from build123d import *

# Parameters (mm, degrees)
F0_R      = 3.25
F1_DEPTH  = 2.5
F2_R      = 1.5
F3_DEPTH  = 2.5
F4_R      = 7
F4_R_2    = 1.5
F5_DEPTH  = 3
F6_R      = 1.5
F7_DEPTH  = 3
F8_W      = 2
F8_H      = 2
F9_DEPTH  = 2
F11_DEPTH = 1


with BuildPart() as f1:
    # F0 (on Top) → F1 (new body)
    with BuildSketch(Plane.XY):
        with Locations((-13.149204, -17.084545)):
            Circle(F0_R)
    extrude(amount=F1_DEPTH)

    # F2 (on face) → F3 (join)
    with BuildSketch(Plane.XY.offset(2.5)):
        with Locations((-13.149204, -17.084545)):
            Circle(F2_R)
    extrude(amount=F3_DEPTH)

    # F4 (on face) → F5 (join)
    with BuildSketch(Plane.XY.offset(5)):
        with Locations((-13.149204, -17.084545)):
            Circle(F4_R)
        with Locations((-13.149204, -17.084545)):
            Circle(F4_R_2, mode=Mode.SUBTRACT)
    extrude(amount=F5_DEPTH)

    # F6 (on face) → F7 (join)
    with BuildSketch(Plane.XY.offset(5)):
        with Locations((-13.149204, -17.084545)):
            Circle(F6_R)
    extrude(amount=F7_DEPTH)

    # F8 (on face) → F9 (join)
    with BuildSketch(Plane.XY.offset(8)):
        with Locations((-16.149204, -14.084545)):
            Rectangle(F8_W, F8_H)
        with Locations((-10.149204, -14.084545)):
            Rectangle(F8_W, F8_H)
        with Locations((-10.149204, -20.084545)):
            Rectangle(F8_W, F8_H)
        with Locations((-16.149204, -20.084545)):
            Rectangle(F8_W, F8_H)
    extrude(amount=F9_DEPTH)

    # F10 (on face) → F11 (join)
    with BuildSketch(Plane.XY.offset(10)):
        Polygon((-9.149204, -13.084545), (-15.149204, -13.084545), (-15.149204, -15.084545), (-17.149204, -15.084545), (-17.149204, -21.084545), (-9.149204, -21.084545), align=None)
    extrude(amount=-F11_DEPTH)


solid = f1.part
Verification items for the finished model (mm, model axes). A direction names the side the tool comes from. Coordinates: 2 decimals unless noted, no trailing zeros. Write each loop counter-clockwise with the first axis right and the second up, starting at its lowest first coordinate (ties: lowest second). Pieces come first, ordered by that corner, then holes. Notation, with made-up numbers: M 79.5,6.25 L 86.5,6.25 A9 cw 86.5,20.25 Z; hole C 37.25,8 d9. An arc over 180 degrees is marked long. Use a Markdown table: item, result.
Q1. Go/stop test with flat-tipped pins: P1, Ø1, axis at y = -20.5, z = 1.5, coming from the +X side; P2, Ø0.5, axis at x = -10, z = 8.5, coming from the -Y side; P3, Ø1.6, axis at y = -16, z = 9, coming from the -X side. Record where each tip stops, or that it passes through.
Reply:
| item | result |
|---|---|
| P1 | stops at x = -11.71 |
| P2 | stops at y = -21.08 |
| P3 | stops at x = -17.15 |
Q2. Sectioned sample at C-C, the plane y = -17.5. Record the boundary of the cut face in (x, z), plus the area to 3 significant figures.
Reply:
| item | result |
|---|---|
| outline | M -20.14,5 L -14.59,5 L -14.59,2.5 L -16.37,2.5 L -16.37,0 L -9.93,0 L -9.93,2.5 L -11.71,2.5 L -11.71,5 L -6.16,5 L -6.16,8 L -20.14,8 Z; M -17.15,9 L -9.15,9 L -9.15,10 L -17.15,10 Z |
| area | 73.2 mm² |
Q3. Draft check along Y on faces 5 (the face through (-16.2, -15.085, 8.5)), 6 (the face through (-15, -18, 2.5)), 7 (the face through (-13.2, -13.085, 9.2)). Enter one of: +Y half, -Y half, draft (parallel to the pull), parting line (faces both ways), or undercut.
Reply:
| item | result |
|---|---|
| face 5 | undercut |
| face 6 | draft |
| face 7 | +Y half |
Q4. Sectioned sample at B-B, the plane x = -16. Record the boundary of the cut face in (y, z).
Reply:
| item | result |
|---|---|
| outline | M -23.48,5 L -10.69,5 L -10.69,8 L -13.08,8 L -13.08,10 L -21.08,10 L -21.08,8 L -23.48,8 Z; M -18.65,0 L -15.52,0 L -15.52,2.5 L -18.65,2.5 Z; hole M -19.08,8 L -15.08,8 L -15.08,9 L -19.08,9 Z |
Q5. Set-up check for faces 1 (the face through (-13.2, -21.085, 9.2)), 2 (the face through (-17.149, -17.1, 9.2)), 3 (the face through (-13, -17, 9)), 4 (the face through (-15.149, -14.1, 8.5)): record each of +Z, -Z, +X, -X, +Y, -Y from which the full face is reachable in a straight line by a thin tool's end or side.
Reply:
| item | result |
|---|---|
| face 1 | +Z, +X, -X, -Y |
| face 2 | +Z, -X, +Y, -Y |
| face 3 | none |
| face 4 | +Y, -Y |
Q6. Thickness scan on line 1 (Z direction, x = -11.75, y = -18); line 2 (Z direction, x = -10.75, y = -20); line 3 (Z direction, x = -18, y = -18). Record the ranges inside material, lowest first.
Reply:
| item | result |
|---|---|
| line 1 | z = 0 to 2.5, 5 to 8, 9 to 10 |
| line 2 | z = 5 to 10 |
| line 3 | z = 5 to 8 |
Q7. Sectioned sample at A-A, the plane y = -14.5. Record the boundary of the cut face in (x, z), plus the area to 3 significant figures.
Reply:
| item | result |
|---|---|
| outline | M -19.65,5 L -6.64,5 L -6.64,8 L -9.15,8 L -9.15,10 L -17.15,10 L -17.15,8 L -19.65,8 Z; M -15.12,0 L -11.18,0 L -11.18,2.5 L -15.12,2.5 Z; hole M -15.15,8 L -11.15,8 L -11.15,9 L -15.15,9 Z |
| area | 60.9 mm² |
Q8. Sectioned sample at D-D, the plane x = -12. Record the boundary of the cut face in (y, z), plus the area to 3 significant figures.
Reply:
| item | result |
|---|---|
| outline | M -23.99,5 L -18.05,5 L -18.05,2.5 L -20.12,2.5 L -20.12,0 L -14.04,0 L -14.04,2.5 L -16.12,2.5 L -16.12,5 L -10.18,5 L -10.18,8 L -23.99,8 Z; M -21.08,9 L -13.08,9 L -13.08,10 L -21.08,10 Z |
| area | 69.5 mm² |
